Design review of the part built by this model. Coordinates are the model's own, in mm. Round coordinates to 2 decimals unless told otherwise and drop trailing zeros. Loops run counter-clockwise (first coordinate to the right, second up) from the corner with the lowest first, then second, coordinate; pieces in that order, holes last. Notation, with made-up numbers: M 31,35 L 79,35 A29 ccw 79,74 Z; hole C -1,22 d2. An arc over 180 degrees is marked long. Use a Markdown table: item, result.
from build123d import *

# Parameters (mm, degrees)
SKETCH1_W                = 80
SKETCH1_H                = 138.754765379
BOSS_EXTRUDE1_DEPTH      = 10
FORO_PER_VITE_M8_1_D     = 8.4
SCHIZZO1_R               = 3.25
TAGLIO_ESTRUSIONE1_DEPTH = 2604.992537461
RACCORDO1_R              = 16


with BuildPart() as part:
    # Sketch1 → Boss-Extrude1 (new body)
    with BuildSketch(Plane.XY):
        with Locations((-1780.42117355, -1792.542026427)):
            Rectangle(SKETCH1_W, SKETCH1_H)
    extrude(amount=BOSS_EXTRUDE1_DEPTH)

    # Foro per Vite M8-1 (through all)
    with Locations(Plane.XY.offset(10)):
        with Locations((-1760.42117355, -1841.919409116), (-1800.42117355, -1841.919409116)):
            Hole(FORO_PER_VITE_M8_1_D / 2)

    # Schizzo1 → Taglio-Estrusione1 (cut, through all)
    with BuildSketch(Plane.XY.offset(10)):
        with Locations((-1803.421173548, -1731.919409116)):
            Circle(SCHIZZO1_R)
        with Locations((-1803.421173548, -1749.919409116)):
            Circle(SCHIZZO1_R)
        with Locations((-1757.421173548, -1731.919409116)):
            Circle(SCHIZZO1_R)
        with Locations((-1757.421173548, -1749.919409116)):
            Circle(SCHIZZO1_R)
    extrude(amount=-TAGLIO_ESTRUSIONE1_DEPTH, mode=Mode.SUBTRACT)

    # Raccordo1
    raccordo1_edges = [part.edges().sort_by_distance(p)[0] for p in [
        (-1820.42117355, -1723.164643737, 5),
        (-1740.42117355, -1723.164643737, 5),
    ]]
    fillet(raccordo1_edges, radius=RACCORDO1_R)


solid = part.part
1. Take a section at C-C on x = -1815. Give the boundary of the cut face in (y, z), and give its area (3 significant figures).
Check values:
| item | result |
|---|---|
| outline | M -1861.92,0 L -1727.16,0 L -1727.16,10 L -1861.92,10 Z |
| area | 1,350 mm² |
2. Take a section at A-A on z = 7. Give the boundary of the cut face in (x, y), and give its area (3 significant figures).
Check values:
| item | result |
|---|---|
| outline | M -1820.42,-1861.92 L -1740.42,-1861.92 L -1740.42,-1739.16 A16 ccw -1756.42,-1723.16 L -1804.42,-1723.16 A16 ccw -1820.42,-1739.16 Z; hole C -1803.42,-1749.92 d6.5; hole C -1803.42,-1731.92 d6.5; hole C -1800.42,-1841.92 d8.4; hole C -1760.42,-1841.92 d8.4; hole C -1757.42,-1749.92 d6.5; hole C -1757.42,-1731.92 d6.5 |
| area | 10,700 mm² |
3. Wall thickness on line 1 along Y through (x, z) = (-1760, 0.5); line 2 along X through (y, z) = (-1838.5, 2.75); line 3 along Y through (x, z) = (-1756, 3): over which ranges is each line inside the solid? List them lowest first. Write a range as from..to.
Check values:
| item | result |
|---|---|
| line 1 | y = -1861.92..-1846.1, -1837.74..-1751.9, -1747.94..-1733.9, -1729.94..-1723.16 |
| line 2 | x = -1820.42..-1802.86, -1797.98..-1762.86, -1757.98..-1740.42 |
| line 3 | y = -1861.92..-1752.84, -1747..-1734.84, -1729..-1723.17 |
4. Take a section at B-B on x = -1747. Give the boundary of the cut face in (y, z).
Check values:
| item | result |
|---|---|
| outline | M -1861.92,0 L -1726.23,0 L -1726.23,10 L -1861.92,10 Z |
5. The part is to be moulded in two halves that separate along X. For faces 1 (the face through (-1760.67, -1731.78, 5.07)), 2 (the face through (-1740.421, -1801, 5)), 3 (the face through (-1781, -1861.919, 5)), say which applies: pulls with the +X half, pulls with the -X half, needs draft (parallel to the pull), parting line crosses it, or undercut.
Check values:
| item | result |
|---|---|
| face 1 | undercut |
| face 2 | pulls with the +X half |
| face 3 | needs draft |
6. Insertion check: pin 1 (6 mm diameter, centred on x = -1803.42, y = -1749.92, fed in from -Z). The pin has a flat end and moves straight along its axis. Give the tip position at first contact, or say it passes through.
Check values:
| item | result |
|---|---|
| pin 1 | passes through |
